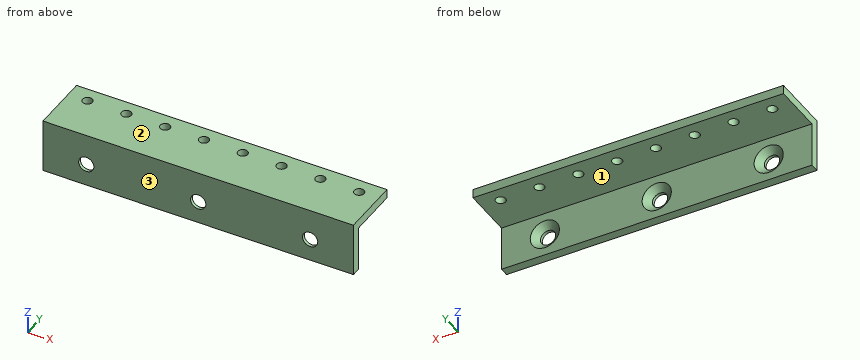
```python
from build123d import *

# Parameters (mm, degrees)
SKETCH2_W                                  = 104
SKETCH2_H                                  = 20
BOSS_EXTRUDE1_DEPTH                        = 3
M4X0_7_TAPPED_HOLE1_D                      = 3.3
SKETCH5_W                                  = 104
SKETCH5_H                                  = 3
BOSS_EXTRUDE2_DEPTH                        = 15
CSK_FOR_10_FLAT_HEAD_MACHINE_SCREW_2_COUNT = 2
CSK_FOR_10_FLAT_HEAD_MACHINE_SCREW_2_PITCH = 37.5
CSK_FOR_10_FLAT_HEAD_MACHINE_SCREW_3_COUNT = 2
CSK_FOR_10_FLAT_HEAD_MACHINE_SCREW_3_PITCH = 75


with BuildPart() as part:
    # Sketch2 → Boss-Extrude1 (new body)
    with BuildSketch(Plane.XY):
        with Locations((0, -10)):
            Rectangle(SKETCH2_W, SKETCH2_H)
    extrude(amount=BOSS_EXTRUDE1_DEPTH)

    # M4x0.7 Tapped Hole1 (through all)
    with Locations(Plane.XY.offset(3)):
        with Locations((-45.5, -5), (45.5, -5), (-32.5, -5), (-19.5, -5), (-6.5, -5), (6.5, -5), (19.5, -5), (32.5, -5)):
            Hole(M4X0_7_TAPPED_HOLE1_D / 2)

    # Sketch5 → Boss-Extrude2 (add)
    with BuildSketch(Plane(origin=(0, 0, 0), x_dir=(-1, 0, 0), z_dir=(0, 0, -1))):
        with Locations((0, -18.5)):
            Rectangle(SKETCH5_W, SKETCH5_H)
    extrude(amount=BOSS_EXTRUDE2_DEPTH)

    # Sketch7 → CSK for #10 Flat Head Machine Screw (100)1 (revolve, cut)
    with BuildSketch(Plane(origin=(37.5, -17, -7.5), x_dir=(0, 0, 1), z_dir=(1, 0, 0))):
        Polygon((0, 0), (0, 3), (2.5527, 3), (2.5527, 1.960808018), (4.8895, 0), align=None)
    csk_for_10_flat_head_machine_screw_100 = revolve(axis=Axis((37.5, -10.65, -7.5), (0, -1, 0)), mode=Mode.SUBTRACT)

    # CSK for _10 Flat Head Machine Screw  2: CSK for #10 Flat Head Machine Screw (100)1 ×2
    with Locations(*[(-i * CSK_FOR_10_FLAT_HEAD_MACHINE_SCREW_2_PITCH, 0, 0) for i in range(1, CSK_FOR_10_FLAT_HEAD_MACHINE_SCREW_2_COUNT)]):
        add(csk_for_10_flat_head_machine_screw_100, mode=Mode.SUBTRACT)

    # CSK for _10 Flat Head Machine Screw  3: CSK for #10 Flat Head Machine Screw (100)1 ×2
    with Locations(*[(-i * CSK_FOR_10_FLAT_HEAD_MACHINE_SCREW_3_PITCH, 0, 0) for i in range(1, CSK_FOR_10_FLAT_HEAD_MACHINE_SCREW_3_COUNT)]):
        add(csk_for_10_flat_head_machine_screw_100, mode=Mode.SUBTRACT)


solid = part.part
```
Here's how the part is built. I have some questions about the finished solid (model axes, mm). Face numbers are marked on the shaded views. Round coordinates to 2 decimals unless told otherwise and drop trailing zeros. Order: outer loops, then holes, each group sorted by start corner. A loop starts at its lowest first (then second) coordinate and runs counter-clockwise, first axis right, second up. Notation, with made-up numbers: (47, -31.75) -> (99, -31.75) arc R20 ccw to (99, -3.75) -> close; hole circle Ø11 at (65, -22). An arc over 180 degrees is marked (long way). Use a Markdown table: item, result. Add a question column.
(1) If we mould it in two halves opening along Z, with no side actions, what happens to the marked faces 1, 2 and 3? For each: released by +Z, released by -Z, zero draft, split by the parting line, or undercut.
(2) Suppose I cut it at C-C, the plane x = 19.5. Please give me the cut outline in (y, z), and give its area (3 significant figures).
(3) Suppose I cut it at D-D, the plane y = -14.5. Please give me the cut outline in (x, z).
(4) For pin 1 Ø4.5 at (x, z) = (0, -7.5) entering from -Y; pin 2 Ø4 at (x, y) = (-19.5, -5) entering from -Z; pin 3 Ø4 at (x, z) = (23.5, -3.5) entering from +Y, each with a flat end and sliding along its axis, tell me the tip position at first contact or that it passes through.
(5) I need wall thicknesses on line 1 along X through (y, z) = (-19.5, -7.5); line 2 along Z through (x, y) = (0, -19.6); line 3 along Y through (x, z) = (32.5, 1.7). Which ranges of each line are inside material? Lowest first, please.
(6) Suppose I cut it at B-B, the plane x = -37.5. Please give me the cut outline in (y, z), and give its area (3 significant figures).
(7) Suppose I cut it at A-A, the plane z = 1. Count the separate pieces of the cut face and the enclosed holes in it, and give its area (3 significant figures).
Verdict:
| question | item | result |
|---|---|---|
| 1 | face 1 | released by -Z |
| 1 | face 2 | released by +Z |
| 1 | face 3 | zero draft |
| 2 | outline | (-20, -15) -> (-17, -15) -> (-17, 0) -> (-6.65, 0) -> (-6.65, 3) -> (-20, 3) -> close; (-3.35, 0) -> (0, 0) -> (0, 3) -> (-3.35, 3) -> close |
| 2 | area | 95.1 mm2 |
| 3 | outline | (-52, 0) -> (52, 0) -> (52, 3) -> (-52, 3) -> close |
| 4 | pin 1 | through |
| 4 | pin 2 | z = 0 |
| 4 | pin 3 | y = -17 |
| 5 | line 1 | -52 to -40.05, -34.95 to -2.55, 2.55 to 34.95, 40.05 to 52 |
| 5 | line 2 | -15 to -10.05, -4.95 to 3 |
| 5 | line 3 | -20 to -6.65, -3.35 to 0 |
| 6 | outline | (-20, -15) -> (-17, -15) -> (-17, -12.39) -> (-18.96, -10.05) -> (-20, -10.05) -> close; (-20, -4.95) -> (-18.96, -4.95) -> (-17, -2.61) -> (-17, 0) -> (0, 0) -> (0, 3) -> (-20, 3) -> close |
| 6 | area | 85.1 mm2 |
| 7 | separate pieces | 1 |
| 7 | enclosed holes | 8 |
| 7 | area | 2,010 mm2 |
